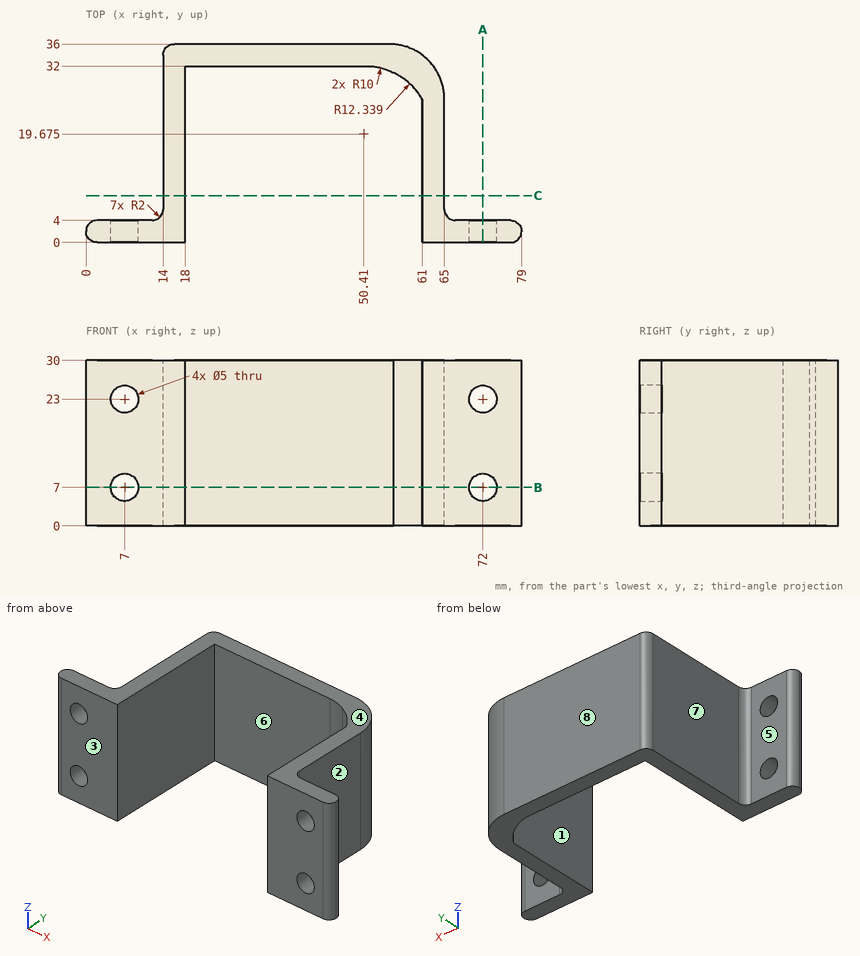
Job drawing, mm, ordinate dimensions from the low corner. One solid piece. A direction names the side the tool comes from. Coordinates: 2 decimals unless noted, no trailing zeros. Order: outer loops, then holes, each group sorted by start corner. A loop starts at its lowest first (then second) coordinate and runs counter-clockwise, first axis right, second up. Notation, with made-up numbers: M 77,20 L 133,20 A25 ccw 133,50 Z; hole C 1,12 d8. An arc over 180 degrees is marked long. Answer as CSV lines item,"result".
(1) Band-saw the part on B-B, the plane z = 7. State how many separate pieces and enclosed holes the cut face has, then the cut area to 3 significant figures.
Geometry says:
separate pieces,"3"
enclosed holes,"0"
area,"526 mm2"
(2) Band-saw the part on C-C, the plane y = 8.5. List the corners of the cut face in (x, z).
Geometry says:
outline,"M 14,0 L 18,0 L 18,30 L 14,30 Z; M 61,0 L 65,0 L 65,30 L 61,30 Z"
(3) Wall check: line 1 along X through (y, z) = (25.5, 13.25); line 2 along X through (y, z) = (1.9, 7); line 3 along X through (y, z) = (1.3, 7). Give the ranges that are in metal, low to high.
Geometry says:
line 1,"x = 14 to 18, 61 to 65"
line 2,"x = 0 to 4.5, 9.5 to 18, 61 to 69.5, 74.5 to 79"
line 3,"x = 0.13 to 4.5, 9.5 to 18, 61 to 69.5, 74.5 to 78.87"
(4) 3-axis set-ups, long thin cutter, end or side, ignore diameter. For the marked faces 1, 2, 3, 4 and 5: which of +Z, -Z, +X, -X, +Y, -Y reach the whole face in a straight line?
Geometry says:
face 1,"+Z, -Z, -Y"
face 2,"+Z, -Z, +X, +Y"
face 3,"+Z, -Z, +X, -X, -Y"
face 4,"+Z, +X, -X, +Y, -Y"
face 5,"+Z, -Z, -X, +Y"
(5) Flat gauge pins, fed straight in: pin 1 (6 mm diameter, centred on x = 72, z = 23, fed in from -Y); pin 2 (6 mm diameter, centred on x = 7, z = 23, fed in from +Y); pin 3 (2 mm diameter, centred on y = 10.5, z = 10.5, fed in from -X); pin 4 (1.5 mm diameter, centred on x = 62, z = 13, fed in from +Y) (1 decimal). Where does each tip first touch, or does it go through?
Geometry says:
pin 1,"stops at y = 0"
pin 2,"stops at y = 4"
pin 3,"stops at x = 14"
pin 4,"stops at y = 33.8"
(6) Band-saw the part on A-A, the plane x = 72. List the corners of the cut face in (y, z).
Geometry says:
outline,"M 0,0 L 4,0 L 4,4.5 L 0,4.5 Z; M 0,9.5 L 4,9.5 L 4,20.5 L 0,20.5 Z; M 0,25.5 L 4,25.5 L 4,30 L 0,30 Z"
(7) Pull direction X, two halves, no side cores. Call the marked faces 6, 7 and 8: +X half, -X half, draft (parallel to the pull), parting line (faces both ways), or undercut.
Geometry says:
face 6,"undercut"
face 7,"-X half"
face 8,"draft"
